The model under review builds one solid part; all positions refer to its coordinate system, in mm. A direction names the side the tool comes from. Coordinates: 2 decimals unless noted, no trailing zeros. Write each loop counter-clockwise with the first axis right and the second up, starting at its lowest first coordinate (ties: lowest second). Pieces come first, ordered by that corner, then holes.
Autodesk Inventor part; units mm, degrees
ref_plane "YZ Plane" through (0, 0, 0) normal (1, 0, 0) x (0, 1, 0)
ref_plane "XZ Plane" through (0, 0, 0) normal (0, 1, 0) x (-1, 0, 0)
ref_plane "XY Plane" through (0, 0, 0) normal (0, 0, 1) x (1, 0, 0)
sketch "Sketch1" plane through (0, 0, 0) normal (0, 1, 0) x (-1, 0, 0)
  line L0 (48.5, 48.5) -> (-48.5, 48.5)
  line L1 (-48.5, 48.5) -> (-48.5, -48.5)
  line L2 (-48.5, -48.5) -> (48.5, -48.5)
  line L3 (48.5, -48.5) -> (48.5, 48.5)
  point P0 (0, 0)
  point P1 (48.5, 0)
  point P2 (0, -48.5)
  dimension "d0" = 97
  dimension "d1" = 97
extrude "Extrusion1" add sketch "Sketch1" along normal mid plane 5
sketch "Sketch2" plane through (0, -2.5, 0) normal (0, -1, 0) x (1, 0, 0)
  line L0 (-42.865, 37.465) -> (-42.865, -36.195) construction
  line L1 (42.865, 40.005) -> (42.865, -40.005) construction
  line L2 (-42.865, 6.4948) -> (42.865, 6.4948) construction
  point P0 (0, 0)
  point P1 (42.865, 0)
  point P2 (0, 6.4948)
  dimension "d4" = 73.66
  dimension "d5" = 80.01
  dimension "d6" = 85.73
  dimension "d7" = 3.81
hole "Hole1" at (-42.865, -2.5, 37.465) at (42.865, -2.5, 40.005) at (-42.865, -2.5, -36.195) at (42.865, -2.5, -40.005) direction (0, 1, 0) diameter 3.6 end through all
chamfer "Chamfer1" distance 5 angle 45 4 edges at (48.5, 0, -48.5) (-48.5, 0, -48.5) (48.5, 0, 48.5) (-48.5, 0, 48.5)
sketch "Sketch3" plane through (48.5, -2.5, 43.5) normal (1, 0, 0) x (0, 0, -1)
  point P0 (43.5, 2.5)
  point P1 (71, 2.5)
  point P2 (16, 2.5)
  dimension "d18" = 55
  dimension "d19" = 27.5
hole "Hole2" at (48.5, 0, -27.5) at (48.5, 0, 27.5) direction (-1, 0, 0) diameter 2.1565 depth 4
pattern_circular "Circular Pattern1" count 4 over 360 about axis through (0, -10, 0) along (0, 1, 0) of "Hole2"
sketch "Sketch5" plane through (0, 2.5, 0) normal (0, 1, 0) x (1, 0, 0)
  line L0 (-15, 25) -> (0, 25)
  line L1 (0, 25) -> (0, -25)
  line L2 (0, -25) -> (-15, -25)
  line L3 (-15, -25) -> (-15, 25)
  point P0 (0, 0)
  point P1 (0, 0)
  dimension "d38" = 15
  dimension "d39" = 50
extrude "Extrusion3" cut sketch "Sketch5" against normal through all
sketch "Sketch6" plane through (0, 2.5, 0) normal (0, 1, 0) x (1, 0, 0)
  line L0 (-48.5, 43.5) -> (-48.5, -43.5)
  line L1 (-43.5, 10) -> (-48.5, 10)
  line L2 (-48.5, 10) -> (-48.5, -10)
  line L3 (-48.5, -10) -> (-43.5, -10)
  line L4 (-43.5, -10) -> (-43.5, 10)
  point P0 (0, 0)
  point P1 (-48.5, 0)
  dimension "d42" = 5
  dimension "d43" = 20
extrude "Extrusion4" cut sketch "Sketch6" against normal through all
pattern_circular "Circular Pattern3" count 4 over 360 about axis through (0, -10, 0) along (0, 1, 0) of "Extrusion4"
sketch "Sketch7" plane through (0, 2.5, 0) normal (0, 1, 0) x (1, 0, 0)
  circle A0 centre (-42.865, -37.465) radius 1.8
  circle A1 centre (-42.865, 36.195) radius 1.8
  circle A2 centre (42.865, 40.005) radius 1.8
  circle A3 centre (42.865, -40.005) radius 1.8
  circle A4 centre (42.865, -18.495) radius 1.8
  line L0 (43.5, -10) -> (43.5, 10)
  circle A5 centre (42.865, 18.495) radius 1.8
  line L1 (-48.5, -28.5782) -> (-48.5, -26.4218)
  circle A6 centre (-33.765, -37.465) radius 1.8
  circle A7 centre (-33.765, 36.195) radius 1.8
  point P0 (0, 0)
extrude "Extrusion5" cut sketch "Sketch7" against normal blind 5 contours A4 | A5 | A6 | A7
sketch "Sketch8" plane through (0, 2.5, 0) normal (0, 1, 0) x (1, 0, 0)
  point P0 (0, 0)
equation "\"d1\" = d0"
properties part number "stackframesupportbottom" material "Aluminum 6061"
Item 1: Take a section at A-A, the plane z = -7. Write out the cut boundary in (x, y), plus the area to 3 significant figures.
Solved:
outline: (-43.5, -2.5) - (-15, -2.5) - (-15, 2.5) - (-43.5, 2.5) - close; (0, -2.5) - (43.5, -2.5) - (43.5, 2.5) - (0, 2.5) - close
area: 360 mm2
Item 2: Take a section at B-B, the plane x = -12. Write out the cut boundary in (y, z).
Solved:
outline: (-2.5, -48.5) - (2.5, -48.5) - (2.5, -25) - (-2.5, -25) - close; (-2.5, 25) - (2.5, 25) - (2.5, 48.5) - (-2.5, 48.5) - close
Item 3: To check wall thickness, follow line 1 along X through (y, z) = (-1.9, 37.5); line 2 along X through (y, z) = (0.3, -15); line 3 along Z through (x, y) = (43, 1.25). State the ranges of each line that lie inside material, in increasing order.
Solved:
line 1: x = -48.5 to -44.66, -41.07 to -35.56, -31.97 to 48.5
line 2: x = -48.5 to -15, 0 to 48.5
line 3: z = -48.5 to -41.8, -38.21 to -20.29, -16.7 to 16.7, 20.29 to 38.21, 41.8 to 48.5
Item 4: Mouldability with a two-part tool opening along Y and no side actions: class faces 1 (the face through (1, 2.5, 1)), 2 (the face through (-7, 0, 25)), 3 (the face through (-44.5, 0, 27)) as pulls with the +Y half, pulls with the -Y half, needs draft (parallel to the pull), parting line crosses it, or undercut.
Solved:
face 1: pulls with the +Y half
face 2: needs draft
face 3: undercut
Item 5: Take a section at C-C, the plane y = 0. Count the separate pieces of the cut face and the enclosed holes in it, plus the area to 3 significant figures.
Solved:
separate pieces: 1
enclosed holes: 9
area: 8,060 mm2
Item 6: Machinability: for faces 4 (the face through (-10, 0, 46)), 5 (the face through (28.577, -0.047, -46.472)), 6 (the face through (0, 0, 0)), which of the approach directions +Z, -Z, +X, -X, +Y, -Y give a long, thin tool a straight path to every point of the face, cutting with its end or side? Answer none if there is none.
Solved:
face 4: +Z, +Y, -Y
face 5: -Z
face 6: +Y, -Y
Item 7: For pin 1 (2.5 mm diameter, centred on y = 0.5, z = 46.5, fed in from -X); pin 2 (1.5 mm diameter, centred on x = 46, y = 0.5, fed in from -Z); pin 3 (0.6 mm diameter, centred on x = 27.5, y = -0.5, fed in from -Z); pin 4 (3 mm diameter, centred on x = 42.865, z = -18.495, fed in from -Y), all flat-tipped, find the tip position at first contact; note any pin that passes through.
Solved:
pin 1: stops at x = -46.75
pin 2: stops at z = -46.75
pin 3: stops at z = -44.5
pin 4: passes through
